Geometry check sheet. Reference: the model listing, model coordinates, mm. Face numbers are marked on the shaded views. A direction names the side the tool comes from. Round coordinates to 2 decimals unless told otherwise and drop trailing zeros. Order: outer loops, then holes, each group sorted by start corner. A loop starts at its lowest first (then second) coordinate and runs counter-clockwise, first axis right, second up.
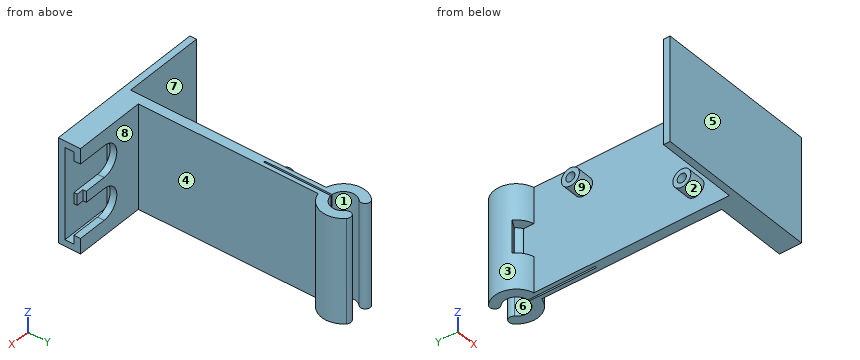
Autodesk Inventor part; units mm, degrees
ref_plane "YZ Plane" through (0, 0, 0) normal (1, 0, 0) x (0, 1, 0)
ref_plane "XZ Plane" through (0, 0, 0) normal (0, 1, 0) x (-1, 0, 0)
ref_plane "XY Plane" through (0, 0, 0) normal (0, 0, 1) x (1, 0, 0)
sketch "Sketch1" plane through (0, 0, 0) normal (0, 1, 0) x (-1, 0, 0)
  line L0 (11, -16) -> (-11, -16)
  line L1 (-11, -16) -> (-11, 16)
  line L2 (-11, 16) -> (11, 16)
  line L3 (11, 16) -> (11, -16)
  line L4 (11, -16) -> (-11, 16) construction
  line L5 (-11, -16) -> (11, 16) construction
  circle A0 centre (-2, 6.5) radius 4.8
  line L6 (-2, 6.5) -> (-2, -6.5)
  circle A1 centre (-2, -6.5) radius 4.8
  line L7 (-2, 11.3) -> (-11, 11.3)
  line L8 (-2, 1.7) -> (-11, 1.7)
  line L9 (-2, -1.7) -> (-11, -1.7)
  line L10 (-2, -11.3) -> (-11, -11.3)
  point P0 (0, 0)
  point P1 (-2, 0)
  dimension "d0" = 22
  dimension "d1" = 32
  dimension "d2" = 9.6
  dimension "d3" = 13
  dimension "d4" = 9.6
extrude "Extrusion1" add sketch "Sketch1" along normal blind 2 contours L0 L1 L10 A1 L6 A0 L7 L2 L3 | L1 L8 L6 L9
sketch "Sketch2" plane through (0, 0, 0) normal (0, -1, 0) x (1, 0, 0)
  line L0 (-11, 16) -> (11, 16)
  line L1 (11, 16) -> (-11, 16)
  line L2 (-11, -16) -> (-11, 16)
  line L3 (-11, 16) -> (-11, -16)
  line L4 (11, -16) -> (-11, -16)
  line L5 (-11, -16) -> (11, -16)
  line L6 (11, -16) -> (11, -14)
  line L7 (11, -11.3) -> (11, -16)
  line L8 (11, -14) -> (-5, -14)
  line L9 (-5, -14) -> (-5, 14)
  line L10 (-5, 14) -> (11, 14)
  line L11 (11, 16) -> (11, 11.3)
  point P0 (0, 0)
  dimension "d7" = 2
  dimension "d8" = 16
  dimension "d9" = 28
extrude "Extrusion2" add sketch "Sketch2" along normal blind 2.75
sketch "Sketch3" plane through (-11, 2, -16) normal (-1, 0, 0) x (0, 0, 1)
  line L0 (0, 0) -> (0, -4.75)
  line L1 (0, -4.75) -> (32, -4.75)
  line L2 (32, -4.75) -> (32, 49.75)
  line L3 (32, 49.75) -> (0, 49.75)
  line L4 (0, 49.75) -> (0, -4.75)
  point P0 (16, -2)
  dimension "d12" = 54.5
extrude "Extrusion3" add sketch "Sketch3" along normal blind 3
sketch "Sketch4" plane through (0, -2.75, 0) normal (0, -1, 0) x (1, 0, 0)
  line L0 (11, 16) -> (11, 11.3)
  line L1 (11, 16) -> (-39, 16)
  line L2 (-39, 16) -> (-39, -16)
  line L3 (-39, -16) -> (11, -16)
  line L4 (11, -16) -> (11, 16)
  point P0 (0, 0)
  dimension "d15" = 50
extrude "Extrusion4" add sketch "Sketch4" along normal blind 2
sketch "Sketch5" plane through (-5, 0, 14) normal (1, 0, 0) x (0, 0, -1)
  line L0 (0, 0) -> (0, -2.75)
  line L1 (30, -2.75) -> (-2, -2.75)
  line L2 (0, 0) -> (2.9896, 0)
  line L3 (2.9896, 0) -> (2.9896, -2.75)
  line L4 (2.9896, -2.75) -> (0, -2.5)
  line L5 (0, -2.5) -> (0, 0)
  point P0 (14, 0)
  dimension "d18" = 3
extrude "Extrusion5" cut sketch "Sketch5" against normal up to surface (9 mm away)
sketch "Sketch6" plane through (11, 0, 1.7) normal (1, 0, 0) x (0, 0, -1)
  line L0 (0, 0) -> (0, 2)
  line L1 (3.4, 0) -> (3.4, 2)
  line L2 (0, 1) -> (3.4, 1)
  line L3 (3.4, 1) -> (3.4, 2)
  line L4 (3.4, 2) -> (0, 2)
  line L5 (0, 2) -> (0, 1)
  point P0 (1.7, 0)
extrude "Extrusion6" cut sketch "Sketch6" against normal blind 2.2
sketch "Sketch8" plane through (-14, 2, -16) normal (-1, 0, 0) x (0, 0, 1)
  circle A0 centre (24.6, 39.75) radius 2.75
  circle A1 centre (24.6, 39.75) radius 1.4
  line L0 (4, 47.25) -> (28, 47.25) construction
  line L1 (28, 47.25) -> (28, -1.75) construction
  line L2 (28, -1.75) -> (4, -1.75) construction
  line L3 (4, -1.75) -> (4, 47.25) construction
  circle A2 centre (7.4, 5.75) radius 2.75
  circle A3 centre (7.4, 5.75) radius 1.4
  line L4 (4, 47.25) -> (28, -1.75) construction
  line L5 (32, -4.75) -> (32, -6.75) construction
  line L6 (32, 49.75) -> (0, 49.75) construction
  line L7 (0, -4.75) -> (32, 49.75) construction
  point P0 (16, -2)
  point P1 (16, 22.75)
  point P2 (16, 22.5)
  dimension "d24" = 5.5
  dimension "d25" = 2.8
  dimension "d26" = 24
  dimension "d27" = 49
  dimension "d28" = 3.4
  dimension "d29" = 7.5
  dimension "d30" = 5.5
  dimension "d31" = 2.8
  dimension "d32" = 3.4
  dimension "d33" = 7.5
extrude "Extrusion7" add sketch "Sketch8" along normal blind 5
sketch "Sketch9" plane through (0, 0, 0) normal (0, 0, 1) x (1, 0, 0)
  line L0 (-14, -2.75) -> (-14, 51.75)
  line L1 (-12.5, 56.75) -> (-12.5, 54.25) construction
  line L2 (-12.25, 56.75) -> (-12.25, 54.25)
  line L3 (-12.25, 54.25) -> (-12.75, 54.25)
  line L4 (-12.75, 54.25) -> (-12.75, 56.75)
  line L5 (-12.75, 56.75) -> (-12.25, 54.25) construction
  line L6 (-12.25, 56.75) -> (-12.75, 54.25) construction
  circle A0 centre (-12.5, 63.45) radius 3.7
  circle A1 centre (-12.5, 63.45) radius 6.7
  line L7 (-12.5, 63.45) -> (-12.5, 56.75) construction
  line L8 (-12.25, 56.75) -> (-12.25, 59.7585)
  line L9 (-12.25, 59.7585) -> (-12.75, 59.7585)
  line L10 (-12.75, 59.7585) -> (-12.75, 56.75)
  line L11 (-12.75, 59.7585) -> (-12.25, 59.7585)
  line L12 (-12.25, 59.7585) -> (-12.25, 70.1453)
  line L13 (-12.25, 70.1453) -> (-12.75, 70.1453)
  line L14 (-12.75, 70.1453) -> (-12.75, 59.7585)
  line L15 (-12.5, 63.45) -> (-5.8, 63.45) construction
  line L16 (-12.5, 63.45) -> (-5.8, 63.45) construction
  line L17 (-7.7624, 68.1876) -> (-9.8837, 66.0663) construction
  line L18 (-17.2376, 68.1876) -> (-15.1163, 66.0663) construction
  circle A2 centre (-16.177, 67.127) radius 1.5
  circle A3 centre (-8.823, 67.127) radius 1.5
  line L19 (-11, 51.75) -> (-14, 51.75)
  line L20 (-14, 51.75) -> (-11, 51.75)
  line L21 (-11, 51.75) -> (-11, 56.75)
  line L22 (-11, 56.75) -> (-14, 56.75)
  line L23 (-14, 56.75) -> (-14, 51.75)
  line L24 (-14, 56.75) -> (-11, 56.75)
  line L25 (-11, 56.75) -> (-11, 56.9201)
  line L26 (-11, 56.9201) -> (-14, 56.9201)
  line L27 (-14, 56.9201) -> (-14, 56.75)
  point P0 (0, 0)
  point P1 (-12.5, 55.5)
  point P2 (-17.2376, 68.1876)
  point P3 (-12.75, 56.7547)
  point P4 (-12.25, 56.7547)
  point P5 (-7.7624, 68.1876)
  dimension "d47" = 0.5
  dimension "d48" = 7.4
  dimension "d49" = 13.4
  dimension "d50" = 5
extrude "Extrusion8" add sketch "Sketch9" along normal mid plane 32 contours L22 L21 L19 L23 L4 L3 L2 | L8 A1 L25 L22 | L8 L26 A1 | L26 L8 A0 A3 A1 | L10 L22 L27 A1 | A1 L26 L10 | L26 A1 A2 A0 L10 | A3 | A2
sketch "Sketch10" plane through (-11, 2, 16) normal (0, 0, 1) x (1, 0, 0)
  line L0 (-1.75, 52.25) -> (-1.25, 52.25)
  line L1 (-1.75, 52.25) -> (-1.25, 52.25)
  line L2 (-1.25, 52.25) -> (-1.25, 37.25)
  line L3 (-1.25, 37.25) -> (-1.75, 37.25)
  line L4 (-1.75, 37.25) -> (-1.75, 52.25)
  point P0 (11, -2)
  dimension "d51" = 15
extrude "Extrusion9" cut sketch "Sketch10" against normal through all
sketch "Sketch11" plane through (0, 0, 0) normal (0, 0, 1) x (1, 0, 0)
  line L0 (-14, -2.75) -> (-14, 56.9201)
  line L1 (-14, 56.9201) -> (-14, 60.0677)
  arc A0 (-15.1163, 66.0663) -> (-12.75, 59.7585) centre (-12.5, 63.45) ccw
  line L2 (-12.5, 63.45) -> (-18.3024, 60.1)
  arc A1 (-17.2376, 68.1876) -> (-14, 56.9201) centre (-12.5, 63.45) ccw
  point P0 (0, 0)
  point P1 (-15.7043, 61.6)
  dimension "d56" = 60
extrude "Extrusion10" cut sketch "Sketch11" along normal mid plane 10
properties part number "prototype_8_1_3DPrint"
(1) Sectioned sample at C-C, the plane z = -8.6. Record the cut outline in (x, y).
Returned:
outline: (-39, -4.75) - (11, -4.75) - (11, -2.75) - (-5, -2.75) - (-5, 0) - (-2.32, 0) - (-2.32, 2) - (-11, 2) - (-11, 56.92) arc R6.7 ccw to (-7.76, 68.19) arc R1.5 ccw to (-9.88, 66.07) arc R3.7 cw to (-12.25, 59.76) - (-12.25, 39.25) - (-12.75, 39.25) - (-12.75, 59.76) arc R3.7 cw to (-15.12, 66.07) arc R1.5 ccw to (-17.24, 68.19) arc R6.7 ccw to (-14, 56.92) - (-14, 10.5) - (-19, 10.5) - (-19, 9.15) - (-14, 9.15) - (-14, 6.35) - (-19, 6.35) - (-19, 5) - (-14, 5) - (-14, -2.75) - (-39, -2.75) - close
(2) Sectioned sample at D-D, the plane x = -35.5. Record the cut outline in (y, z), and give its area (3 significant figures).
Returned:
outline: (-4.75, -16) - (-2.75, -16) - (-2.75, 16) - (-4.75, 16) - close
area: 64.0 mm2
(3) Set-up check for the marked faces 5, 6, 7, 8 and 9: record each of +Z, -Z, +X, -X, +Y, -Y from which the full face is reachable in a straight line by a thin tool's end or side.
Returned:
face 5: +Z, -Z, +X, -X, -Y
face 6: +Z, -Z
face 7: none
face 8: +Z, -Z, +X
face 9: -X
(4) Sectioned sample at B-B, the plane z = 12.5. Record the cut outline in (x, y), and give its area (3 significant figures).
Returned:
outline: (-39, -4.75) - (11, -4.75) - (11, -2.75) - (-39, -2.75) - close; (-17.24, 68.19) arc R6.7 ccw to (-14, 56.92) - (-14, 0) - (11, 0) - (11, 2) - (-11, 2) - (-11, 56.92) arc R6.7 ccw to (-7.76, 68.19) arc R1.5 ccw to (-9.88, 66.07) arc R3.7 cw to (-12.25, 59.76) - (-12.25, 39.25) - (-12.75, 39.25) - (-12.75, 59.76) arc R3.7 cw to (-15.12, 66.07) arc R1.5 ccw to start
area: 385 mm2
(5) Material ranges on line 1 (X direction, y = 48.5, z = 1.5); line 2 (Y direction, x = 5, z = -0.5); line 3 (Y direction, x = -17.05, z = -8.6), recorded low to high.
Returned:
line 1: x = -14 to -12.75, -12.25 to -11
line 2: y = -4.75 to -2.75, 0 to 2
line 3: y = -4.75 to -2.75, 5 to 6.35, 9.15 to 10.5, 58.53 to 68.35
(6) Draft check along X on the marked faces 1, 2, 3 and 4. Enter one of: released by +X, released by -X, zero draft, split by the parting line, or undercut.
Returned:
face 1: undercut
face 2: zero draft
face 3: released by -X
face 4: released by +X
(7) Depth check by flat-ended pin: P1, Ø8, axis at y = 24, z = -7.5, coming from the -X side; P2, Ø1.7, axis at y = 41.75, z = 8.6, coming from the +X side; P3, Ø2, axis at y = -0.5, z = -5.5, coming from the +X side; P4, Ø1.1, axis at y = 1.5, z = 0, coming from the +X side. Enter the tip coordinate at first touch or a pass-through.
Returned:
P1: stops at x = -14
P2: stops at x = -11
P3: stops at x = -2.42
P4: stops at x = 11
(8) Sectioned sample at A-A, the plane y = 7.75. Record the cut outline in (x, z).
Returned:
outline: (-19, -11.35) - (-14, -11.35) - (-14, -16) - (-11, -16) - (-11, 16) - (-14, 16) - (-14, -5.85) - (-19, -5.85) - (-19, -7.2) - (-14, -7.2) - (-14, -10) - (-19, -10) - close
